The listing builds one solid part. Answer for the finished solid, in the listing's coordinates (mm). A direction names the side the tool comes from. Round coordinates to 2 decimals unless told otherwise and drop trailing zeros. Write each loop counter-clockwise with the first axis right and the second up, starting at its lowest first coordinate (ties: lowest second). Pieces come first, ordered by that corner, then holes.
(1) A cutting plane is placed at D-D, the plane x = 9.5. Give the vertices of the cut face in (y, z).
(2) For faces 1 (the face through (-11, 10, -54.398)), 2 (the face through (-3, 10, -79)), 3 (the face through (15.3, 17, -1)), 4 (the face through (5, 10, -65.398)), determine the directions among +Z, -Z, +X, -X, +Y, -Y from which every point of the face is accessible in a straight line to the end or side of a thin tool.
(3) A cutting plane is placed at B-B, the plane x = -11. Give the vertices of the cut face in (y, z), and give its area (3 significant figures).
(4) Each of these flat-tipped pins is pushed along its axis until it touches: pin 1 Ø4 at (y, z) = (3.5, -0.5) entering from -X; pin 2 Ø6 at (y, z) = (13.5, -13.5) entering from +X; pin 3 Ø2.5 at (y, z) = (10, -76.4) entering from -X; pin 4 Ø5 at (x, y) = (-3.5, 29) entering from -Z. Where does it stop, or does it pass through?
(5) A cutting plane is placed at C-C, the plane y = 6.5. Give the vertices of the cut face in (x, z).
(6) Find the intervals of material crossed by probe 1 along Z at (x, y) = (-10.75, 30); probe 2 along Y at (x, z) = (5, -50.5); probe 3 along X at (y, z) = (14, 2), in increasing order.
(7) A cutting plane is placed at A-A, the plane y = 25. Give the vertices of the cut face in (x, z), and give its area (3 significant figures).
(8) The mould has two halves that part along Z. Classify faces 5 (the face through (-0.07, 12.291, 19.273)), 6 (the face through (0, 20, -23)), 7 (the face through (-0.07, 11.906, 27.793)), 8 (the face through (0, 10, -84.398)): +Z half, -Z half, draft (parallel to the pull), parting line (faces both ways), or undercut.
from build123d import *

# Parameters (mm, degrees)
BOSS_EXTRU_1_DEPTH      = 20
ESQUISSE3_R             = 1.5
ENL_V_MAT_EXTRU_3_DEPTH = 20
ESQUISSE4_R             = 1.5
ENL_V_MAT_EXTRU_4_DEPTH = 10
ESQUISSE5_R             = 1.5
ENL_V_MAT_EXTRU_5_DEPTH = 10
ESQUISSE6_R             = 1.4
BOSS_EXTRU_2_DEPTH      = 10.3


with BuildPart() as part:
    # Esquisse1 → Boss.-Extru.1 (new body)
    with BuildSketch(Plane(origin=(0, 0, 0), x_dir=(1, 0, 0), z_dir=(0, 1, 0))):
        with BuildLine():
            Line((-3, 84.398281038), (-3, 69.398281038))
            Line((-3, 69.398281038), (-7, 69.398281038))
            Line((-7, 69.398281038), (-7, 65.398281038))
            Line((-7, 65.398281038), (-3, 65.398281038))
            Line((-3, 65.398281038), (-3, 54.398281038))
            Line((-3, 54.398281038), (-18.71, 54.398281038))
            ThreePointArc((-18.71, 54.398281038), (-22.308577777, 49.499317693), (-26.183329952, 44.81574006))
            ThreePointArc((-26.183329952, 44.81574006), (-12.83252844, 48.159570073), (-5, 36.842476876))
            Line((-5, 36.842476876), (-5, -39.182739587))
            Line((-5, -39.182739587), (0, -39.182739587))
            Line((0, -39.182739587), (0, 84.398281038))
            Line((0, 84.398281038), (-3, 84.398281038))
        make_face()
    boss_extru_1 = extrude(amount=BOSS_EXTRU_1_DEPTH)

    # Symétrie1: Boss.-Extru.1 across plane
    add(boss_extru_1.mirror(Plane(origin=(0, 20, -84.398281038), x_dir=(0, 0, 1), z_dir=(-1, 0, 0))))

    # Esquisse3 → Enlèv. mat.-Extru.3 (cut)
    with BuildSketch(Plane.ZY.offset(3)):
        with Locations((-76.398281038, 10)):
            Circle(ESQUISSE3_R)
        with Locations((-60.398281038, 10)):
            Circle(ESQUISSE3_R)
    extrude(amount=-ENL_V_MAT_EXTRU_3_DEPTH, mode=Mode.SUBTRACT)

    # Esquisse4 → Enlèv. mat.-Extru.4 (cut)
    with BuildSketch(Plane.ZY.offset(5)):
        with Locations((29.291975875, 11.84)):
            Circle(ESQUISSE4_R)
    extrude(amount=-ENL_V_MAT_EXTRU_4_DEPTH, mode=Mode.SUBTRACT)

    # Esquisse5 → Enlèv. mat.-Extru.5 (cut)
    with BuildSketch(Plane.ZY.offset(5)):
        with Locations((17.841975875, 11.84)):
            Circle(ESQUISSE5_R)
    extrude(amount=-ENL_V_MAT_EXTRU_5_DEPTH, mode=Mode.SUBTRACT)

    # Esquisse6 → Boss.-Extru.2 (add)
    with BuildSketch(Plane(origin=(5, 0, 0), x_dir=(0, 0, -1), z_dir=(1, 0, 0))):
        with BuildLine():
            Line((5.308208853, 0), (-2.691791147, 0))
            Line((-2.691791147, 0), (-2.691791147, 30))
            ThreePointArc((-2.691791147, 30), (1.308208853, 34), (5.308208853, 30))
            Line((5.308208853, 30), (5.308208853, 0))
        make_face()
        with Locations(Location((1.308208853, 30, 0), (0, 0, 180))):
            Circle(ESQUISSE6_R, mode=Mode.SUBTRACT)
    boss_extru_2 = extrude(amount=BOSS_EXTRU_2_DEPTH)

    # Symétrie2: Boss.-Extru.2 across plane
    add(boss_extru_2.mirror(Plane.ZY))


solid = part.part
Solutions:
1. outline: (0, -54.4) - (20, -54.4) - (20, -46.25) - (0, -46.25) - close; (0, -5.31) - (30, -5.31) arc R4 ccw to (30, 2.69) - (0, 2.69) - close; hole circle Ø2.8 at (30, -1.31)
2. face 1: -X, +Y, -Y
2. face 2: -Z, -X, +Y, -Y
2. face 3: +Z, +X, +Y, -Y
2. face 4: +X, +Y, -Y
3. outline: (0, -54.4) - (20, -54.4) - (20, -47.29) - (0, -47.29) - close; (0, -5.31) - (30, -5.31) arc R4 ccw to (30, 2.69) - (0, 2.69) - close; hole circle Ø2.8 at (30, -1.31)
3. area: 401 mm2
4. pin 1: stops at x = -15.3
4. pin 2: stops at x = 5
4. pin 3: passes through
4. pin 4: stops at z = -5.31
5. outline: (-26.18, -44.82) arc R105.5 cw to (-18.71, -54.4) - (-3, -54.4) - (-3, -65.4) - (-7, -65.4) - (-7, -69.4) - (-3, -69.4) - (-3, -84.4) - (3, -84.4) - (3, -69.4) - (7, -69.4) - (7, -65.4) - (3, -65.4) - (3, -54.4) - (18.71, -54.4) arc R105.5 cw to (26.18, -44.82) arc R12.09 cw to (5, -36.84) - (5, -5.31) - (15.3, -5.31) - (15.3, 2.69) - (5, 2.69) - (5, 39.18) - (-5, 39.18) - (-5, 2.69) - (-15.3, 2.69) - (-15.3, -5.31) - (-5, -5.31) - (-5, -36.84) arc R12.09 cw to start
6. probe 1: z = -5.31 to -2.71, 0.09 to 2.69
6. probe 2: y = 0 to 20
6. probe 3: x = -15.3 to 15.3
7. outline: (-15.3, -5.31) - (-5, -5.31) - (-5, 2.69) - (-15.3, 2.69) - close; (5, -5.31) - (15.3, -5.31) - (15.3, 2.69) - (5, 2.69) - close
7. area: 165 mm2
8. face 5: undercut
8. face 6: draft
8. face 7: undercut
8. face 8: -Z half
